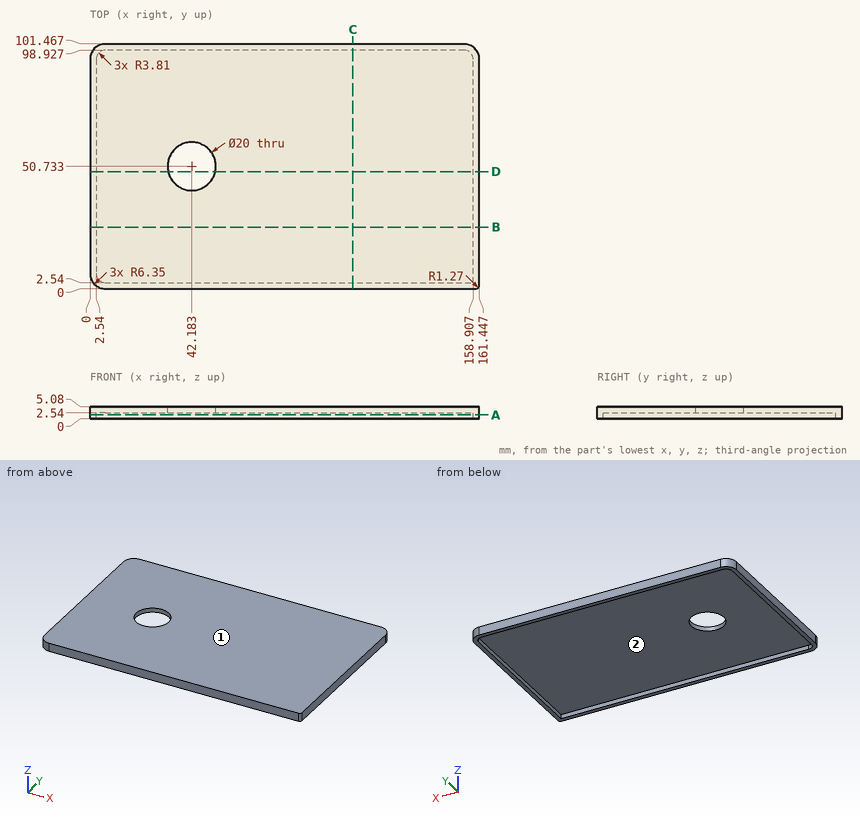
The figure shows three views and two pictorial views of one solid part (mm, origin at its lowest corner). Answer the questions. Coordinates: 2 decimals unless noted, no trailing zeros. Order: outer loops, then holes, each group sorted by start corner. A loop starts at its lowest first (then second) coordinate and runs counter-clockwise, first axis right, second up. Notation, with made-up numbers: (13.5, 12.5) - (51.5, 12.5) arc R30 ccw to (51.5, 43.5) - close; hole circle Ø3 at (54.5, -12). An arc over 180 degrees is marked (long way). Answer as a JSON object with one key per item and string values.
1. Consider line 1 (X direction, y = 87.5, z = 0.75); line 2 (Y direction, x = 41.5, z = 2.35); line 3 (Z direction, x = 147.5, y = 68). Determine where each line is inside the solid, lowest interval first.
Output values:
{"line 1": "x = 0 to 2.54, 158.91 to 161.45", "line 2": "y = 0 to 2.54, 98.93 to 101.47", "line 3": "z = 2.54 to 5.08"}
2. Find section D-D on y = 48.5. Determine the outline of the cut face in (x, z) (1 decimal).
Output values:
{"outline": "(0, 0) - (2.5, 0) - (2.5, 2.5) - (32.4, 2.5) - (32.4, 5.1) - (0, 5.1) - close; (51.9, 2.5) - (158.9, 2.5) - (158.9, 0) - (161.4, 0) - (161.4, 5.1) - (51.9, 5.1) - close"}
3. This flat-tipped pin is pushed along its axis until it touches: P1, Ø1.5, axis at y = 64, z = 4, coming from the -X side. Where does it stop, or does it pass through?
Output values:
{"P1": "stops at x = 0"}
4. Find section A-A on z = 1.7. Determine the outline of the cut face in (x, y), plus the area to 3 significant figures.
Output values:
{"outline": "(0, 6.35) arc R6.35 ccw to (6.35, 0) - (160.18, 0) arc R1.27 ccw to (161.45, 1.27) - (161.45, 95.12) arc R6.35 ccw to (155.1, 101.47) - (6.35, 101.47) arc R6.35 ccw to (0, 95.12) - close; hole (2.54, 6.35) arc R3.81 ccw to (6.35, 2.54) - (158.91, 2.54) - (158.91, 95.12) arc R3.81 ccw to (155.1, 98.93) - (6.35, 98.93) arc R3.81 ccw to (2.54, 95.12) - close", "area": "1,290 mm²"}
5. Find section B-B on y = 25.5. Determine the outline of the cut face in (x, z).
Output values:
{"outline": "(0, 0) - (2.54, 0) - (2.54, 2.54) - (158.91, 2.54) - (158.91, 0) - (161.45, 0) - (161.45, 5.08) - (0, 5.08) - close"}
6. The mould has two halves that part along X. Classify the marked faces 1 and 2: +X half, -X half, draft (parallel to the pull), parting line (faces both ways), or undercut.
Output values:
{"face 1": "draft", "face 2": "undercut"}
7. Find section C-C on x = 109. Determine the outline of the cut face in (y, z).
Output values:
{"outline": "(0, 0) - (2.54, 0) - (2.54, 2.54) - (98.93, 2.54) - (98.93, 0) - (101.47, 0) - (101.47, 5.08) - (0, 5.08) - close"}
